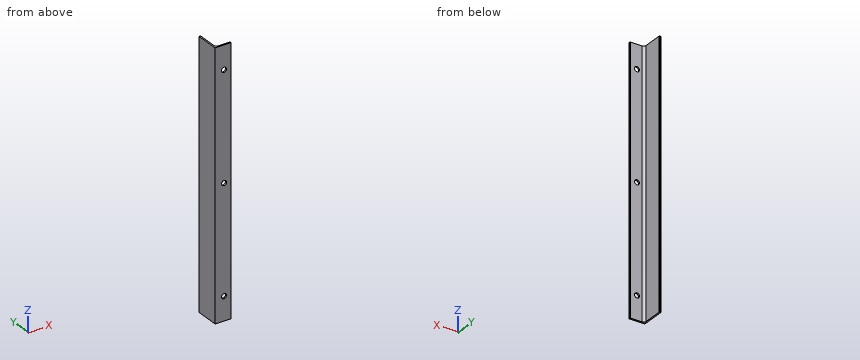
Autodesk Inventor part; units mm, degrees
ref_plane "Start plane" through (0, 0, 0) normal (0, 0, 1) x (1, 0, 0)
ref_plane "End plane" through (0, 0, 844.55) normal (0, 0, 1) x (1, 0, 0)
ref_plane "YZ Plane" through (0, 0, 0) normal (1, 0, 0) x (0, 1, 0)
ref_plane "Start plane" through (0, 0, 0) normal (0, 0, 1) x (1, 0, 0)
ref_plane "End plane" through (0, 0, 844.55) normal (0, 0, 1) x (1, 0, 0)
sketch "Sketch" plane through (0, 0, 0) normal (0, 0, 1) x (1, 0, 0)
  line L0 (0, 76.2) -> (0, 0)
  line L1 (0, 0) -> (50.8, 0)
  line L2 (50.8, 0) -> (50.8, 2.7625)
  line L3 (48.8, 4.7625) -> (12.6365, 4.7625)
  line L4 (4.7625, 12.6365) -> (4.7625, 74.2)
  line L5 (2.7625, 76.2) -> (0, 76.2)
  line L6 (-7.0414, 0) -> (21.5385, 0) construction
  line L7 (0, -8.0414) -> (0, 34.5385) construction
  arc A0 (4.7625, 12.6365) -> (12.6365, 4.7625) centre (12.6365, 12.6365) ccw
  arc A1 (50.8, 2.7625) -> (48.8, 4.7625) centre (48.8, 2.7625) ccw
  arc A2 (4.7625, 74.2) -> (2.7625, 76.2) centre (2.7625, 74.2) ccw
  line L8 (0, 93.5453) -> (0, -24.9725) construction
  line L9 (-18.6925, 0) -> (62.8653, 0) construction
  point P0 (50.8, 4.7625)
  point P1 (4.7625, 4.7625)
  point P2 (4.7625, 76.2)
  dimension "d12" = 4.7625
  dimension "d13" = 76.2
  dimension "d14" = 50.8
  dimension "d15" = 0
  dimension "d16" = 4.7625
  dimension "d17" = 0
  dimension "d18" = 7.874
  dimension "d19" = 2
extrude "Body" add sketch "Sketch" along normal up to surface (844.55 mm away) from surface at 0
sketch "Sketch4" plane through (0, 0, 0) normal (0, 0, 1) x (1, 0, 0)
  line L0 (0, 0) -> (10, 0)
ref_plane "Work Plane3" through (0, 0, 0) normal (0, -1, 0) x (1, 0, 0)
sketch "Sketch5" plane through (0, 0, 0) normal (0, -1, 0) x (1, 0, 0)
  line L0 (-2, 0) -> (12, 0)
  line L1 (-2, 844.55) -> (12, 844.55)
  dimension "d37" = 844.55
sketch "Sketch3" plane through (0, 0, 0) normal (0, -1, 0) x (1, 0, 0)
  line L0 (50.8, 844.55) -> (0, 844.55)
  line L1 (50.8, 0) -> (50.8, 844.55)
  line L2 (28.6513, 844.55) -> (28.6513, 0)
  point P0 (28.6513, 422.275)
  point P1 (50.8, 422.275)
  point P2 (28.6513, 768.35)
  point P3 (28.6513, 76.2)
  point P4 (28.6513, 422.275)
  dimension "d22" = 844.55
  dimension "d23" = 76.2
  dimension "d24" = 422.275
  dimension "d25" = 768.35
  dimension "d26" = 76.2
  dimension "d27" = 422.275
  dimension "d28" = 768.35
hole "Hole1" at (28.6513, 0, 768.35) at (28.6513, 0, 76.2) at (28.6513, 0, 422.275) direction (0, 1, 0) diameter 15.875 end through all
equation "\"d12\" = G_T"
equation "\"d13\" = G_H"
equation "\"d14\" = G_W"
equation "\"d16\" = G_T"
equation "\"d18\" = G_IR"
equation "\"d4\" = G_L"
equation "\"G_W\" = 50.8"
equation "\"G_H\" = 76.2"
equation "\"G_T\" = 4.7625"
equation "\"G_ER\" = 4.064"
equation "\"G_IR\" = 7.874"
equation "\"G_L\" = d37"
equation "\"ex\" = 0"
equation "\"ey\" = 0"
equation "\"G_OFFSET_START\" = 0"
equation "\"G_OFFSET_END\" = 0"
equation "\"d21\" = G_OFFSET_END + B_L"
equation "\"B_L\" = 844.55"
properties part number "ANSI L 3 x 2 x 3_16 00000005"
For this review, take the finished solid that the model builds, in its own axes (mm). Round coordinates to 2 decimals unless told otherwise and drop trailing zeros. Write each loop counter-clockwise with the first axis right and the second up, starting at its lowest first coordinate (ties: lowest second). Pieces come first, ordered by that corner, then holes. Notation, with made-up numbers: (-39.5, -38.75) - (-29.5, -38.75) arc R16 ccw to (-29.5, -30.75) - close; hole circle Ø11 at (31, -20.5). An arc over 180 degrees is marked (long way). Put each result on its own line as item: value.
Q1. Insertion check: pin 1 Ø4 at (x, z) = (30.5, 641) entering from +Y; pin 2 Ø4 at (x, z) = (9.5, 704.5) entering from +Y; pin 3 Ø14.5 at (x, z) = (28.65, 76.2) entering from +Y; pin 4 Ø18.5 at (y, z) = (48, 327) entering from +X. Each pin has a flat end and moves straight along its axis. Give the tip position at first contact, or say it passes through.
Solved:
pin 1: stops at y = 4.76
pin 2: stops at y = 6.67
pin 3: passes through
pin 4: stops at x = 4.76
Q2. We need section C-C (y = 25). Give the boundary of the cut face in (x, z).
Solved:
outline: (0, 0) - (4.76, 0) - (4.76, 844.55) - (0, 844.55) - close
Q3. Wall thickness on probe 1 along X at (y, z) = (1.2, 768.35); probe 2 along X at (y, z) = (37.5, 582.5): over which ranges is each line inside the solid? List them lowest first.
Solved:
probe 1: x = 0 to 20.71, 36.59 to 50.8
probe 2: x = 0 to 4.76
Q4. We need section A-A (z = 768.35). Give the boundary of the cut face in (x, y).
Solved:
outline: (0, 0) - (20.71, 0) - (20.71, 4.76) - (12.64, 4.76) arc R7.87 cw to (4.76, 12.64) - (4.76, 74.2) arc R2 ccw to (2.76, 76.2) - (0, 76.2) - close; (36.59, 0) - (50.8, 0) - (50.8, 2.76) arc R2 ccw to (48.8, 4.76) - (36.59, 4.76) - close
Q5. We need section B-B (z = 142). Give the boundary of the cut face in (x, y).
Solved:
outline: (0, 0) - (50.8, 0) - (50.8, 2.76) arc R2 ccw to (48.8, 4.76) - (12.64, 4.76) arc R7.87 cw to (4.76, 12.64) - (4.76, 74.2) arc R2 ccw to (2.76, 76.2) - (0, 76.2) - close
